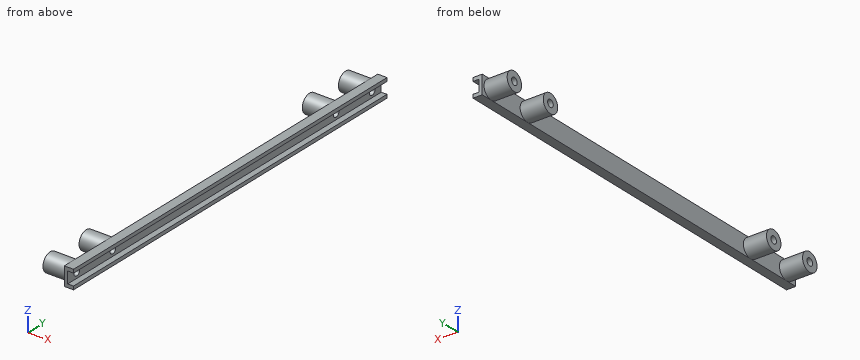
Autodesk Inventor part; units mm, degrees
ref_plane "YZ Plane" through (0, 0, 0) normal (1, 0, 0) x (0, 1, 0)
ref_plane "XZ Plane" through (0, 0, 0) normal (0, 1, 0) x (-1, 0, 0)
ref_plane "XY Plane" through (0, 0, 0) normal (0, 0, 1) x (1, 0, 0)
sketch "Sketch1" plane through (0, 0, 0) normal (0, 1, 0) x (-1, 0, 0)
  line L0 (0, 3.1877) -> (3.1877, 3.1877)
  line L1 (3.1877, 3.1877) -> (3.1877, -3.1877)
  line L2 (3.1877, -3.1877) -> (0, -3.1877)
  line L3 (0, 5.08) -> (5.08, 5.08)
  line L4 (5.08, 5.08) -> (5.08, -5.08)
  line L5 (5.08, -5.08) -> (0, -5.08)
  line L6 (0, -5.08) -> (0, -3.1877)
  line L7 (0, 3.1877) -> (0, 5.08)
  point P0 (0, 0)
  dimension "d0" = 3.1877
  dimension "d1" = 6.3754
  dimension "d2" = 5.08
  dimension "d3" = 10.16
extrude "Extrusion1" add sketch "Sketch1" along normal blind 220.5736
sketch "Sketch2" plane through (-5.08, 0, -5.08) normal (-1, 0, 0) x (0, 0, 1)
  circle A0 centre (5.08, 6.35) radius 1.9844
  circle A1 centre (5.08, 214.2236) radius 1.9844
  circle A2 centre (5.08, 31.75) radius 1.9844
  circle A3 centre (5.08, 188.8236) radius 1.9844
  point P0 (5.08, 0)
  dimension "d6" = 3.9688
  dimension "d7" = 3.9688
  dimension "d12" = 3.9688
  dimension "d13" = 3.9688
sketch "Sketch3" plane through (-5.08, 0, -5.08) normal (-1, 0, 0) x (0, 0, 1)
  point P0 (5.08, 0)
extrude "Extrusion4" cut sketch "Sketch2" against normal blind 12.7
sketch "Sketch5" plane through (-5.08, 6.35, 0) normal (-1, 0, 0) x (0, 0, 1)
  circle A0 centre (0, 0) radius 1.9844
  circle A1 centre (0, 25.4) radius 1.9844
  circle A2 centre (0, 182.4736) radius 1.9844
  circle A3 centre (0, 207.8736) radius 1.9844
  circle A4 centre (0, 0) radius 5.08
  line L0 (-5.08, -6.35) -> (-5.08, 214.2236)
  circle A5 centre (0, 25.4) radius 5.08
  circle A6 centre (0, 207.8736) radius 5.08
  circle A7 centre (0, 182.4736) radius 5.08
  point P0 (0, -6.35)
extrude "Extrusion5" add sketch "Sketch5" along normal blind 12.7
properties part number "hs_intake_front_brace"
Source: CAD feature listing. Evaluate the final solid. Frame: model axes, mm. Round coordinates to 2 decimals unless told otherwise and drop trailing zeros. Loops run counter-clockwise (first coordinate to the right, second up) from the corner with the lowest first, then second, coordinate; pieces in that order, holes last. Notation, with made-up numbers: (67, 29) - (96, 29) arc R15 cw to (96, 42) - close; hole circle Ø10 at (71, 6). An arc over 180 degrees is marked (long way). Write item = value, one per line. Start each with the question number.
(1) Ray query, line 1 along Y through (x, z) = (-5.5, 4.5); line 2 along X through (y, z) = (37.5, -4.25); line 3 along Y through (x, z) = (-9, -3.5). Return the intervals inside material, ascending. Write a range as from..to.
(2) Section query A-A, the plane x = -7.5. Output: boundary loops of the cut face in (y, z).
(3) Section query B-B, the plane y = 201. Output: boundary loops of the cut face in (x, z), plus the area to 3 significant figures.
(4) Pin query (flat end, axial travel): pin 1 (3 mm diameter, centred on x = -14.5, z = -4, fed in from +Y); pin 2 (3 mm diameter, centred on y = 104, z = 0.5, fed in from -X). Return the tip coordinate at first contact, or that it passes through.
(5) Section query C-C, the plane z = 0. State how many separate pieces and enclosed holes the cut face has, plus the area to 3 significant figures.
Conclusion:
q1.line_1 = 3.99..8.71, 29.39..34.11, 186.47..191.18, 211.87..216.58
q1.line_2 = -5.08..0
q1.line_3 = 2.67..10.03, 28.07..35.43, 185.14..192.51, 210.54..217.91
q2.outline = circle Ø10.16 at (6.35, 0); circle Ø10.16 at (31.75, 0); circle Ø10.16 at (188.82, 0); circle Ø10.16 at (214.22, 0); hole circle Ø3.97 at (6.35, 0); hole circle Ø3.97 at (31.75, 0); hole circle Ø3.97 at (188.82, 0); hole circle Ø3.97 at (214.22, 0)
q3.outline = (-5.08, -5.08) - (0, -5.08) - (0, -3.19) - (-3.19, -3.19) - (-3.19, 3.19) - (0, 3.19) - (0, 5.08) - (-5.08, 5.08) - close
q3.area = 31.3 mm2
q4.pin_1 = 218.65
q4.pin_2 = -5.08
q5.separate_pieces = 5
q5.enclosed_holes = 0
q5.area = 702 mm2
